Here's how the part is built. I have some questions about the finished solid (model axes, mm). A direction names the side the tool comes from. Give positions to 0.01 mm unless a question says otherwise; leave off trailing zeros. Loops run counter-clockwise (first coordinate to the right, second up) from the corner with the lowest first, then second, coordinate; pieces in that order, holes last. Notation, with made-up numbers: M 68.5,60.5 L 75.5,60.5 A18 ccw 75.5,71.5 Z; hole C 57.5,68 d8. An arc over 180 degrees is marked long. Answer as CSV lines item,"result". Start each with the question number.
Item 1: For faces 4 (the cylindrical face through (-14, -2.03, -15.57)), 5 (the flat face through (17, -14, -18)), 6 (the flat face through (18, -14, 17)), 7 (the flat face through (-17, -14, 18)), which set-ups out of +Z, -Z, +X, -X, +Y, -Y let a thin tool reach every point of the face, with its end or its side?
Item 2: If we mould it in two halves opening along X, with no side actions, what happens to faces 1 (the cylindrical face through (-14, -2.03, 15.43)), 2 (the cylindrical face through (2.38, 0.94, -10.74)), 3 (the flat face through (-21, -24, 0))? For each: released by +X, released by -X, zero draft, split by the parting line, or undercut.
Item 3: If I drill on line 1 along Z through (x, y) = (15.5, -2.35); line 2 along Y through (x, z) = (-4, 7.5), over which ranges is the centre line in solid material (lowest first)? Write a range as from..to.
Item 4: I want a section at D-D on z = -18. List the corners of the cut face in (x, y) for me.
Item 5: I want a section at A-A on z = 0. List the corners of the cut face in (x, y) for me.
Item 6: Will these pins go through, and if not, where does the flat tip stop? P1, Ø1.8, axis at x = 15.5, z = 15.5, coming from the +Y side; P2, Ø12, axis at x = -7.5, z = -11, coming from the +Y side; P3, Ø0.9, axis at x = 0.5, y = 16, coming from the +Z side; P4, Ø8, axis at y = -17, z = -14.5, coming from the +X side.
Item 7: I want a section at B-B on y = -7. List the corners of the cut face in (x, z) for me.
from build123d import *

# Parameters (mm, degrees)
SKETCH_1_W                = 8
SKETCH_1_H                = 42
EXTRUDE_1_DEPTH           = 0.2
EXTRUDE_2_DEPTH           = 41.6
SKETCH_3_W                = 42
SKETCH_3_H                = 8
EXTRUDE_3_DEPTH           = 0.2
SKETCH_4_W                = 42
SKETCH_4_H                = 42
EXTRUDE_4_DEPTH           = 9
SKETCH_5_R                = 11
EXTRUDE_5_DEPTH           = 1.9
SKETCH_6_R                = 2.5
EXTRUDE_6_DEPTH           = 22.1
CUT_EXTRUDE_1_DEPTH       = 21
SKETCH_8_W                = 2.5
SKETCH_8_H                = 8
HOLE_WIZARD_5_0_5_1_D     = 5
HOLE_WIZARD_5_0_5_1_DEPTH = 5
HOLE_WIZARD_3_0_3_1_D     = 3
HOLE_WIZARD_3_0_3_1_DEPTH = 4
CHAMFER_1_SIZE            = 6.6
CHAMFER_2_SIZE            = 4


with BuildPart() as part:
    # 스케치1 → 보스-돌출1 (new body)
    with BuildSketch(Plane(origin=(-21, 0, 0), x_dir=(0, -1, 0), z_dir=(-1, 0, 0))):
        with Locations((4, 0)):
            Rectangle(SKETCH_1_W, SKETCH_1_H)
    extrude(amount=-EXTRUDE_1_DEPTH)

    # 스케치2 → 보스-돌출2 (add)
    with BuildSketch(Plane(origin=(-20.8, 0, 0), x_dir=(0, 0, -1), z_dir=(1, 0, 0))):
        Polygon((20.8, -8), (20.8, -20), (-20.8, -20), (-20.8, -8), (-21, -8), (-21, 0), (21, 0), (21, -8), align=None)
    extrude(amount=EXTRUDE_2_DEPTH)

    # 스케치3 → 보스-돌출3 (add)
    with BuildSketch(Plane(origin=(20.8, 0, 0), x_dir=(0, 0, -1), z_dir=(1, 0, 0))):
        with Locations((0, -4)):
            Rectangle(SKETCH_3_W, SKETCH_3_H)
    extrude(amount=EXTRUDE_3_DEPTH)

    # 스케치4 → 보스-돌출4 (add)
    with BuildSketch(Plane(origin=(0, -20, 0), x_dir=(1, 0, 0), z_dir=(0, 1, 0))):
        Rectangle(SKETCH_4_W, SKETCH_4_H)
    extrude(amount=-EXTRUDE_4_DEPTH)

    # 스케치5 → 보스-돌출5 (add)
    with BuildSketch(Plane(origin=(0, 0, 0), x_dir=(-1, 0, 0), z_dir=(0, 1, 0))):
        Circle(SKETCH_5_R)
    extrude(amount=EXTRUDE_5_DEPTH)

    # 스케치6 → 보스-돌출6 (add)
    with BuildSketch(Plane(origin=(0, 1.9, 0), x_dir=(-1, 0, 0), z_dir=(0, 1, 0))):
        Circle(SKETCH_6_R)
    extrude(amount=EXTRUDE_6_DEPTH)

    # 스케치7 → 컷-돌출1 (cut)
    with BuildSketch(Plane(origin=(0, 24, 0), x_dir=(-1, 0, 0), z_dir=(0, 1, 0))):
        with BuildLine():
            Line((-1.5, 2), (1.5, 2))
            ThreePointArc((1.5, 2), (0, 2.5), (-1.5, 2))
        make_face()
    extrude(amount=-CUT_EXTRUDE_1_DEPTH, mode=Mode.SUBTRACT)

    # 스케치8 → 컷-회전1 (revolve, cut)
    with BuildSketch(Plane.XY):
        with Locations((1.25, -4)):
            Rectangle(SKETCH_8_W, SKETCH_8_H)
    revolve(axis=Axis((0, 0, 0), (0, -1, 0)), mode=Mode.SUBTRACT)

    # Ø5.0 (5) 지름 구멍1
    with Locations(Plane(origin=(0, -29, 0), x_dir=(-1, 0, 0), z_dir=(0, -1, 0))):
        with Locations((0, 0)):
            Hole(HOLE_WIZARD_5_0_5_1_D / 2, depth=HOLE_WIZARD_5_0_5_1_DEPTH)

    # Ø3.0 (3) 지름 구멍1
    with Locations(Plane(origin=(0, 0, 0), x_dir=(1, 0, 0), z_dir=(0, 1, 0))):
        with Locations((-15.5, 15.5), (15.5, -15.5), (15.5, 15.5), (-15.5, -15.5)):
            Hole(HOLE_WIZARD_3_0_3_1_D / 2, depth=HOLE_WIZARD_3_0_3_1_DEPTH)

    # 모따기1
    chamfer_1_edges = [part.edges().sort_by_distance(p)[0] for p in [
        (-20.8, -14, 20.8),
        (-20.8, -14, -20.8),
        (20.8, -14, 20.8),
        (20.8, -14, -20.8),
    ]]
    chamfer(chamfer_1_edges, length=CHAMFER_1_SIZE)

    # 모따기2
    chamfer_2_edges = [part.edges().sort_by_distance(p)[0] for p in [
        (21, -4, -21),
        (21, -4, 21),
        (-21, -24.5, 21),
        (-21, -24.5, -21),
        (21, -24.5, -21),
        (21, -24.5, 21),
        (-21, -4, 21),
        (-21, -4, -21),
    ]]
    chamfer(chamfer_2_edges, length=CHAMFER_2_SIZE)


solid = part.part
Result:
1,face 4,"+Y"
1,face 5,"-Z, +X"
1,face 6,"+Z, +X"
1,face 7,"+Z, -X"
2,face 1,"undercut"
2,face 2,"split by the parting line"
2,face 3,"released by -X"
3,line 1,"-21..-17, -14..14, 17..21"
3,line 2,"-29..1.9"
4,outline,"M -20,-29 L 20,-29 L 20,-20 L 17,-20 L 17,-8 L 20,-8 L 20,0 L -20,0 L -20,-8 L -17,-8 L -17,-20 L -20,-20 Z"
5,outline,"M -21,-29 L -2.5,-29 L -2.5,-24 L 2.5,-24 L 2.5,-29 L 21,-29 L 21,-20 L 20.8,-20 L 20.8,-8 L 21,-8 L 21,0 L 11,0 L 11,1.9 L 2.5,1.9 L 2.5,24 L -2.5,24 L -2.5,1.9 L -11,1.9 L -11,0 L -21,0 L -21,-8 L -20.8,-8 L -20.8,-20 L -21,-20 Z; hole M -2.5,-8 L 2.5,-8 L 2.5,0 L -2.5,0 Z"
6,P1,"y = -4"
6,P2,"y = 1.9"
6,P3,"z = 2"
6,P4,"x = 21"
7,outline,"M -21,-17 L -17,-21 L 17,-21 L 21,-17 L 21,17 L 17,21 L -17,21 L -21,17 Z; hole C 0,0 d5"
